from build123d import *

# Parameters (mm, degrees)
SKETCH_R   = 1.65
SKETCH_R_2 = 11.5
SKETCH_R_3 = 1.6
PAD_DEPTH  = 2.5
FILLET_R   = 4.5


with BuildPart() as part:
    # Sketch → Pad (new body)
    with BuildSketch(Plane.XY):
        Polygon((20, 20), (-20, 20), (-27.5, 20), (-27.5, -20), (-20, -20), (20, -20), (32, -20), (32, 20), align=None)
        with Locations((-15.5, 15.5)):
            Circle(SKETCH_R, mode=Mode.SUBTRACT)
        with Locations((15.5, 15.5)):
            Circle(SKETCH_R, mode=Mode.SUBTRACT)
        with Locations((15.5, -15.5)):
            Circle(SKETCH_R, mode=Mode.SUBTRACT)
        with Locations((-15.5, -15.5)):
            Circle(SKETCH_R, mode=Mode.SUBTRACT)
        Circle(SKETCH_R_2, mode=Mode.SUBTRACT)
        with Locations((-23.5, 15.5)):
            Circle(SKETCH_R_3, mode=Mode.SUBTRACT)
        with Locations((-23.5, -15.5)):
            Circle(SKETCH_R_3, mode=Mode.SUBTRACT)
        with Locations((28, 15.5)):
            Circle(SKETCH_R_3, mode=Mode.SUBTRACT)
        with Locations((28, -15.5)):
            Circle(SKETCH_R_3, mode=Mode.SUBTRACT)
    extrude(amount=PAD_DEPTH)

    # Fillet
    fillet_edges = [part.edges().sort_by_distance(p)[0] for p in [
        (32, -20, 1.25),
        (32, 20, 1.25),
        (-27.5, 20, 1.25),
        (-27.5, -20, 1.25),
    ]]
    fillet(fillet_edges, radius=FILLET_R)


solid = part.part
The model under review builds one solid part; all positions refer to its coordinate system, in mm. Give positions to 0.01 mm unless a question says otherwise; leave off trailing zeros. Write each loop counter-clockwise with the first axis right and the second up, starting at its lowest first coordinate (ties: lowest second). Pieces come first, ordered by that corner, then holes.
1. Draft analysis for pull direction Y (two halves, no side actions). For faces 1 (the cylindrical face through (30.647, 18.717, 1.268)), 2 (the flat face through (8, 9, 2.5)), 3 (the cylindrical face through (-13.926, -15.004, 1.232)), state which applies: +Y half, -Y half, draft (parallel to the pull), parting line (faces both ways), or undercut.
2. Add section A-A, the plane x = -15.5. Write out the cut boundary in (y, z), plus the area to 3 significant figures.
3. Wall thickness on L1, parallel to Y at x = 15.5, z = 0.75; L2, parallel to Y at x = -24.5, z = 1.35; L3, parallel to X at y = -16, z = 1.3: over which ranges is each line inside the solid? List them lowest first.
4. Add section B-B, the plane x = 0. Write out the cut boundary in (y, z), plus the area to 3 significant figures.
5. Add section D-D, the plane y = -8.5. Write out the cut boundary in (x, z).
6. Add section C-C, the plane z = 1.2. Count the separate pieces of the cut face and the enclosed holes in it, plus the area to 3 significant figures.
Worked answers:
1. face 1: +Y half
1. face 2: draft
1. face 3: undercut
2. outline: (-20, 0) - (-17.15, 0) - (-17.15, 2.5) - (-20, 2.5) - close; (-13.85, 0) - (13.85, 0) - (13.85, 2.5) - (-13.85, 2.5) - close; (17.15, 0) - (20, 0) - (20, 2.5) - (17.15, 2.5) - close
2. area: 83.5 mm2
3. L1: y = -20 to -17.15, -13.85 to 13.85, 17.15 to 20
3. L2: y = -19.74 to -16.75, -14.25 to 14.25, 16.75 to 19.74
3. L3: x = -27.47 to -25.02, -21.98 to -17.07, -13.93 to 13.93, 17.07 to 26.48, 29.52 to 31.97
4. outline: (-20, 0) - (-11.5, 0) - (-11.5, 2.5) - (-20, 2.5) - close; (11.5, 0) - (20, 0) - (20, 2.5) - (11.5, 2.5) - close
4. area: 42.5 mm2
5. outline: (-27.5, 0) - (-7.75, 0) - (-7.75, 2.5) - (-27.5, 2.5) - close; (7.75, 0) - (32, 0) - (32, 2.5) - (7.75, 2.5) - close
6. separate pieces: 1
6. enclosed holes: 9
6. area: 1,880 mm2
